```python
from build123d import *

# Parameters (mm, degrees)
SKETCH_R         = 4.615
EXTRUDE_DEPTH    = 13.65
SKETCH001_W      = 10.4
SKETCH001_H      = 6.9
SKETCH001_R      = 1.6
EXTRUDE001_DEPTH = 2.6


with BuildPart() as body_main:
    # Sketch → Extrude (new body, symmetric)
    with BuildSketch(Plane.YZ):
        with BuildLine():
            Line((-5.5, 14.8), (5.5, 14.8))
            ThreePointArc((5.760824, 14.2224), (5.633177, 14.512448), (5.5, 14.8))
            Line((4.878487, 13.741903), (5.760824, 14.2224))
            ThreePointArc((5.099264, 13.188869), (4.991522, 13.466442), (4.878487, 13.741903))
            Line((6.069929, 13.448108), (5.099264, 13.188869))
            ThreePointArc((6.278586, 12.849682), (6.177122, 13.149894), (6.069929, 13.448108))
            Line((5.357169, 12.449197), (6.278586, 12.849682))
            ThreePointArc((5.528111, 11.878788), (5.44537, 12.164811), (5.357169, 12.449197))
            Line((6.517918, 12.051062), (5.528111, 11.878788))
            ThreePointArc((6.672768, 11.436511), (6.598284, 11.744528), (6.517918, 12.051062))
            Line((5.719511, 11.119185), (6.672768, 11.436511))
            ThreePointArc((5.839274, 10.53588), (5.782184, 10.828106), (5.719511, 11.119185))
            Line((6.840447, 10.619837), (5.839274, 10.53588))
            ThreePointArc((6.940275, 9.993989), (6.893357, 10.307391), (6.840447, 10.619837))
            Line((5.962664, 9.762314), (6.940275, 9.993989))
            ThreePointArc((6.03031, 9.170696), (5.999319, 9.466829), (5.962664, 9.762314))
            Line((7.034984, 9.165675), (6.03031, 9.170696))
            ThreePointArc((7.079005, 8.533446), (7.06002, 8.849771), (7.034984, 9.165675))
            Line((6.08472, 8.389243), (7.079005, 8.533446))
            ThreePointArc((6.099716, 7.793958), (6.095067, 8.091672), (6.08472, 8.389243))
            Line((7.1, 7.7), (6.099716, 7.793958))
            Line((7.1, 7.7), (7.1, 6.95))
            Line((7.1, 6.95), (6.1, 6.85))
            Line((6.1, 6.85), (6.1, 6.1))
            Line((6.1, 6.1), (7.1, 6))
            Line((7.1, 6), (7.1, 5.25))
            Line((7.1, 5.25), (6.1, 5.15))
            Line((6.1, 5.15), (6.1, 4.4))
            Line((6.1, 4.4), (7.1, 4.3))
            Line((7.1, 4.3), (7.1, 3.55))
            Line((7.1, 3.55), (6.1, 3.45))
            Line((6.1, 3.45), (6.1, 2.7))
            Line((6.1, 2.7), (7.1, 2.6))
            Line((7.1, 2.6), (7.1, 0))
            Line((7.1, 0), (-7.1, 0))
            Line((-7.1, 0), (-7.1, 2.6))
            Line((-7.1, 2.6), (-6.1, 2.7))
            Line((-6.1, 2.7), (-6.1, 3.45))
            Line((-6.1, 3.45), (-7.1, 3.55))
            Line((-7.1, 3.55), (-7.1, 4.3))
            Line((-7.1, 4.3), (-6.1, 4.4))
            Line((-6.1, 4.4), (-6.1, 5.15))
            Line((-6.1, 5.15), (-7.1, 5.25))
            Line((-7.1, 5.25), (-7.1, 6))
            Line((-7.1, 6), (-6.1, 6.1))
            Line((-6.1, 6.1), (-6.1, 6.85))
            Line((-6.1, 6.85), (-7.1, 6.95))
            Line((-7.1, 6.95), (-7.1, 7.7))
            Line((-7.1, 7.7), (-6.099716, 7.793958))
            ThreePointArc((-6.08472, 8.389243), (-6.095067, 8.091672), (-6.099716, 7.793958))
            Line((-6.08472, 8.389243), (-7.079005, 8.533446))
            ThreePointArc((-7.034984, 9.165675), (-7.06002, 8.849771), (-7.079005, 8.533446))
            Line((-7.034984, 9.165675), (-6.03031, 9.170696))
            ThreePointArc((-5.962664, 9.762314), (-5.999319, 9.466829), (-6.03031, 9.170696))
            Line((-5.962664, 9.762314), (-6.940275, 9.993989))
            ThreePointArc((-6.840447, 10.619837), (-6.893357, 10.307391), (-6.940275, 9.993989))
            Line((-6.840447, 10.619837), (-5.839274, 10.53588))
            ThreePointArc((-5.719511, 11.119185), (-5.782184, 10.828106), (-5.839274, 10.53588))
            Line((-5.719511, 11.119185), (-6.672768, 11.436511))
            ThreePointArc((-6.517918, 12.051062), (-6.598284, 11.744528), (-6.672768, 11.436511))
            Line((-6.517918, 12.051062), (-5.528111, 11.878788))
            ThreePointArc((-5.357169, 12.449197), (-5.44537, 12.164811), (-5.528111, 11.878788))
            Line((-5.357169, 12.449197), (-6.278586, 12.849682))
            ThreePointArc((-6.069929, 13.448108), (-6.177122, 13.149894), (-6.278586, 12.849682))
            Line((-6.069929, 13.448108), (-5.099264, 13.188869))
            ThreePointArc((-4.878487, 13.741903), (-4.991522, 13.466442), (-5.099264, 13.188869))
            Line((-4.878487, 13.741903), (-5.760824, 14.2224))
            ThreePointArc((-5.5, 14.8), (-5.633177, 14.512448), (-5.760824, 14.2224))
        make_face()
        with Locations((0, 7.7)):
            Circle(SKETCH_R, mode=Mode.SUBTRACT)
    extrude(amount=EXTRUDE_DEPTH, both=True)


with BuildPart() as body:
    # Sketch001 → Extrude001 (new body)
    with BuildSketch(Plane.XY):
        with Locations((8.45, 10.55)):
            Rectangle(SKETCH001_W, SKETCH001_H)
        with Locations((9.15, 9.9)):
            Circle(SKETCH001_R, mode=Mode.SUBTRACT)
        with Locations((-8.45, -10.55)):
            Rectangle(SKETCH001_W, SKETCH001_H)
        with Locations((-9.15, -9.9)):
            Circle(SKETCH001_R, mode=Mode.SUBTRACT)
    extrude(amount=EXTRUDE001_DEPTH)

    # Fusion: union Body Main
    add(body_main.part)


solid = body.part
```
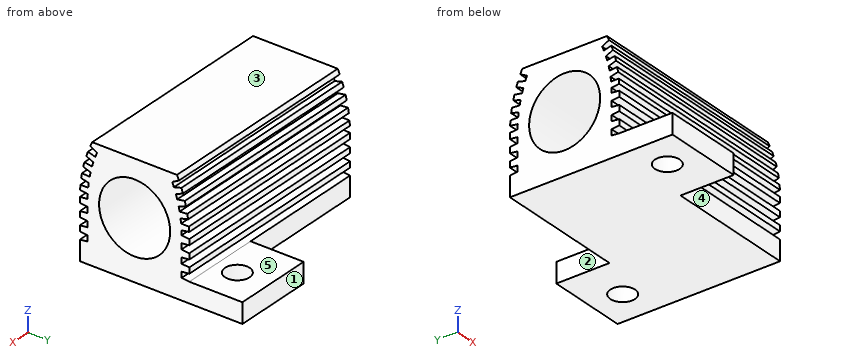
For this review, take the finished solid that the model builds, in its own axes (mm). Face numbers are marked on the shaded views. A direction names the side the tool comes from. Round coordinates to 2 decimals unless told otherwise and drop trailing zeros. Write each loop counter-clockwise with the first axis right and the second up, starting at its lowest first coordinate (ties: lowest second). Pieces come first, ordered by that corner, then holes. Notation, with made-up numbers: (45, -26.5) -> (101, -26.5) arc R23 ccw to (101, 2.5) -> close; hole circle Ø5 at (85.5, -6.75). An arc over 180 degrees is marked (long way). One line per question, with ' | ' between items. Start each with the question number.
(1) Tool access review of the marked faces 1, 2, 3, 4 and 5: name each direction out of +Z, -Z, +X, -X, +Y, -Y from which nothing blocks a thin tool from reaching the whole face with its end or side.
(2) Insertion check: P1, Ø0.8, axis at x = 6, z = 4, coming from the +Y side; P2, Ø0.6, axis at x = 2, z = 4.5, coming from the -Y side; P3, Ø3, axis at y = -9, z = 2, coming from the +X side; P4, Ø3, axis at x = -9.15, y = -9.9, coming from the -Z side. Each pin has a flat end and moves straight along its axis. Give the tip position at first contact, or say it passes through.
(3) Add section C-C, the plane x = 9.15. Give the number of separate pieces and of enclosed holes in the cut face, plus the area to 3 significant figures.
(4) For line 1 along Y through (x, z) = (9.15, 1.6); line 2 along Z through (x, y) = (-2.5, 0) (3 decimals); line 3 along Y through (x, z) = (-9.15, 1.15), list the stretches that pass through material, from the lowest coordinate up. Write a range as from..to.
(5) Add section B-B, the plane z = 4.75. Write out the cut boundary in (x, y), plus the area to 3 significant figures.
(6) Add section A-A, the plane y = 0. Write out the cut boundary in (x, z) (3 decimals).
Answer list:
1) face 1: +Z, -Z, +X, -X, +Y | face 2: +Z, -Z, -X, +Y | face 3: +Z, +X, -X, +Y, -Y | face 4: +Z, -Z, +X, -Y | face 5: +Z, +X, -X, +Y
2) P1: y = 7.1 | P2: y = -7.1 | P3: x = -3.25 | P4: through
3) separate pieces: 2 | enclosed holes: 1 | area: 133 mm²
4) line 1: -7.1..8.3, 11.5..14 | line 2: 0..3.085, 12.315..14.8 | line 3: -14..-11.5, -8.3..7.1
5) outline: (-13.65, -6.1) -> (13.65, -6.1) -> (13.65, -3.55) -> (-13.65, -3.55) -> close; (-13.65, 3.55) -> (13.65, 3.55) -> (13.65, 6.1) -> (-13.65, 6.1) -> close | area: 139 mm²
6) outline: (-13.65, 0) -> (13.65, 0) -> (13.65, 3.085) -> (-13.65, 3.085) -> close; (-13.65, 12.315) -> (13.65, 12.315) -> (13.65, 14.8) -> (-13.65, 14.8) -> close
